Can you work these out from the model? Positions are in its coordinate system, mm. A direction names the side the tool comes from. Give positions to 0.01 mm unless a question says otherwise; leave off trailing zeros. Order: outer loops, then holes, each group sorted by start corner. A loop starts at its lowest first (then second) coordinate and runs counter-clockwise, first axis right, second up.
Item 1: Which directions (+Z, -Z, +X, -X, +Y, -Y) give clear straight access to the entire face, cutting with the end or side of a thin tool? Please do faces 4 (the flat face through (3.2, -8.1, 7)), 5 (the flat face through (4.4, -5, 5)), 6 (the cylindrical face through (-5.158, -3.955, 0.493)).
Item 2: If we mould it in two halves opening along Y, with no side actions, what happens to faces 1 (the cylindrical face through (-2.38, -10.74, 3.45)), 2 (the cylindrical face through (4.57, 7.167, 0.493)), 3 (the flat face through (3.2, -8.1, 0))? For each: +Y half, -Y half, draft (parallel to the pull), parting line (faces both ways), or undercut.
Item 3: I want a section at A-A, the plane y = 0. Write out the boundary of the cut face in (x, z), then the cut area to 3 significant figures.
Item 4: I'm going to push a flat-ended pin straight in: pin 1 Ø1.5 at (x, z) = (-3.5, 1) entering from +Y. Where does the tip first touch, or does it pass through?
Item 5: I want a section at D-D, the plane y = -5.25. Write out the boundary of the cut face in (x, z), then the cut area to 3 significant figures.
Item 6: If I drill on line 1 along Y through (x, z) = (0, 6.05); line 2 along X through (y, z) = (-6, 5.75); line 3 along X through (y, z) = (-3.5, 0.75), over which ranges is the centre line in solid material (lowest first)?
Item 7: I want a section at C-C, the plane x = 7. Write out the boundary of the cut face in (y, z), then the cut area to 3 significant figures.
```python
from build123d import *

# Parameters (mm, degrees)
CYLINDER010_R     = 4
CYLINDER010_DEPTH = 9
CYLINDER009_R     = 6.5
CYLINDER009_DEPTH = 7
CYLINDER012_R     = 5.5
CYLINDER012_DEPTH = 7
CYLINDER011_R     = 9
CYLINDER011_DEPTH = 4
CYLINDER008_R     = 8.5
CYLINDER008_DEPTH = 8
CYLINDER007_R     = 11
CYLINDER007_DEPTH = 7


with BuildPart() as cilindro010:
    # Cylinder010 → Cylinder010 (new body)
    with BuildSketch(Plane.XY.offset(-1)):
        Circle(CYLINDER010_R)
    extrude(amount=CYLINDER010_DEPTH)


with BuildPart() as cut003:
    # Cylinder009 → Cylinder009 (new body)
    with BuildSketch(Plane.XY):
        Circle(CYLINDER009_R)
    extrude(amount=CYLINDER009_DEPTH)

    # Cut003: cut Cilindro010
    add(cilindro010.part, mode=Mode.SUBTRACT)


with BuildPart() as cilindro012:
    # Cylinder012 → Cylinder012 (new body)
    with BuildSketch(Plane.XY):
        Circle(CYLINDER012_R)
    extrude(amount=CYLINDER012_DEPTH)


with BuildPart() as cut004:
    # Cylinder011 → Cylinder011 (new body)
    with BuildSketch(Plane.XY.offset(1)):
        Circle(CYLINDER011_R)
    extrude(amount=CYLINDER011_DEPTH)

    # Cut004: cut Cilindro012
    add(cilindro012.part, mode=Mode.SUBTRACT)


with BuildPart() as cilindro008:
    # Cylinder008 → Cylinder008 (new body)
    with BuildSketch(Plane.XY.offset(-1)):
        Circle(CYLINDER008_R)
    extrude(amount=CYLINDER008_DEPTH)


with BuildPart() as f_608zz:
    # Cylinder007 → Cylinder007 (new body)
    with BuildSketch(Plane.XY):
        Circle(CYLINDER007_R)
    extrude(amount=CYLINDER007_DEPTH)

    # Cut002: cut Cilindro008
    add(cilindro008.part, mode=Mode.SUBTRACT)

    # Fusion003: union Cut003, Cut004
    add(cut003.part)
    add(cut004.part)


solid = f_608zz.part
```
Results list:
1. face 4: +Z, +X, -X, +Y, -Y
1. face 5: +Z
1. face 6: -Z
2. face 1: parting line
2. face 2: undercut
2. face 3: draft
3. outline: (-11, 0) - (-8.5, 0) - (-8.5, 1) - (-6.5, 1) - (-6.5, 0) - (-4, 0) - (-4, 7) - (-6.5, 7) - (-6.5, 5) - (-8.5, 5) - (-8.5, 7) - (-11, 7) - close; (4, 0) - (6.5, 0) - (6.5, 1) - (8.5, 1) - (8.5, 0) - (11, 0) - (11, 7) - (8.5, 7) - (8.5, 5) - (6.5, 5) - (6.5, 7) - (4, 7) - close
3. area: 86.0 mm2
4. pin 1: stops at y = 10.65
5. outline: (-9.67, 0) - (-6.68, 0) - (-6.68, 1) - (-3.83, 1) - (-3.83, 0) - (3.83, 0) - (3.83, 1) - (6.68, 1) - (6.68, 0) - (9.67, 0) - (9.67, 7) - (6.68, 7) - (6.68, 5) - (3.83, 5) - (3.83, 7) - (-3.83, 7) - (-3.83, 5) - (-6.68, 5) - (-6.68, 7) - (-9.67, 7) - close
5. area: 118 mm2
6. line 1: y = -11 to -8.5, -6.5 to -4, 4 to 6.5, 8.5 to 11
6. line 2: x = -9.22 to -6.02, -2.5 to 2.5, 6.02 to 9.22
6. line 3: x = -10.43 to -7.75, -5.48 to -1.94, 1.94 to 5.48, 7.75 to 10.43
7. outline: (-8.49, 0) - (-4.82, 0) - (-4.82, 1) - (4.82, 1) - (4.82, 0) - (8.49, 0) - (8.49, 7) - (4.82, 7) - (4.82, 5) - (-4.82, 5) - (-4.82, 7) - (-8.49, 7) - close
7. area: 89.9 mm2
